Could you check a few things on this model? Use its own coordinates, in mm. Face numbers are marked on the shaded views. A direction names the side the tool comes from. Round coordinates to 2 decimals unless told otherwise and drop trailing zeros. Loops run counter-clockwise (first coordinate to the right, second up) from the corner with the lowest first, then second, coordinate; pieces in that order, holes last.
from build123d import *

# Parameters (mm, degrees)
BOSS_EXTRUDE1_DEPTH = 50
SKETCH2_W           = 7
SKETCH2_H           = 8
BOSS_EXTRUDE2_DEPTH = 50
SKETCH2_3_W         = 7
SKETCH2_3_H         = 8
BOSS_EXTRUDE3_DEPTH = 18
SKETCH3_W           = 10
SKETCH3_H           = 63
SKETCH3_W_2         = 7
SKETCH3_H_2         = 8
BOSS_EXTRUDE4_DEPTH = 82
FILLET1_R           = 5
SKETCH4_W           = 49
SKETCH4_H           = 29.5
CUT_EXTRUDE1_DEPTH  = 63
SKETCH5_W           = 29.5
SKETCH5_H           = 11
BOSS_EXTRUDE5_DEPTH = 49
CUT_EXTRUDE2_DEPTH  = 29.5
SKETCH6_R           = 1.75
CUT_EXTRUDE3_DEPTH  = 5
SKETCH6_6_R         = 0.75
CUT_EXTRUDE4_DEPTH  = 15
SKETCH8_W           = 18
SKETCH8_H           = 9.5
CUT_EXTRUDE5_DEPTH  = 40
SKETCH9_W           = 7
SKETCH9_H           = 9.5
CUT_EXTRUDE6_DEPTH  = 45
SKETCH10_W          = 10
SKETCH10_H          = 10
CUT_EXTRUDE7_DEPTH  = 29.5
SKETCH11_W          = 13
SKETCH11_H          = 48
SKETCH11_H_2        = 7
CUT_EXTRUDE8_DEPTH  = 124.13610356
SKETCH12_W          = 8
SKETCH12_H          = 10
CUT_EXTRUDE9_DEPTH  = 114.279521539
SKETCH13_W          = 10
SKETCH13_H          = 6
CUT_EXTRUDE10_DEPTH = 14
SKETCH15_W          = 14
SKETCH15_H          = 6
CUT_EXTRUDE11_DEPTH = 128.218316291
FILLET2_R           = 3


with BuildPart() as part:
    # Sketch1 → Boss-Extrude1 (new body)
    with BuildSketch(Plane.XY):
        with BuildLine():
            Line((-2.25, -8), (-4.25, -8))
            ThreePointArc((-4.25, -8), (-3.25, -8.5), (-2.25, -8))
        make_face()
        Polygon((10, -25.5), (10, 0), (0, 0), (-18, 0), (-18, -8), (0, -8), (0, -17.5), (-18, -17.5), (-18, -25.5), align=None)
    extrude(amount=BOSS_EXTRUDE1_DEPTH)

    # Sketch2 → Boss-Extrude2 (add)
    with BuildSketch(Plane(origin=(0, 0, 0), x_dir=(0, 0, -1), z_dir=(1, 0, 0))):
        Polygon((7, 0), (0, 0), (0, -8), (2.25, -8), (4.25, -8), (7, -8), align=None)
        Polygon((0, -8), (0, 0), (-10, 0), (-10, -25.5), (0, -25.5), (0, -17.5), align=None)
        with Locations((3.5, -21.5)):
            Rectangle(SKETCH2_W, SKETCH2_H)
        with BuildLine():
            Line((4.25, -8), (2.25, -8))
            ThreePointArc((2.25, -8), (3.25, -8.5), (4.25, -8))
        make_face()
    extrude(amount=BOSS_EXTRUDE2_DEPTH)

    # Sketch2<3> → Boss-Extrude3 (add)
    with BuildSketch(Plane(origin=(0, 0, 0), x_dir=(0, 0, -1), z_dir=(1, 0, 0))):
        Polygon((7, 0), (0, 0), (0, -8), (2.25, -8), (4.25, -8), (7, -8), align=None)
        with Locations((3.5, -21.5)):
            Rectangle(SKETCH2_3_W, SKETCH2_3_H)
    extrude(amount=-BOSS_EXTRUDE3_DEPTH)

    # Sketch3 → Boss-Extrude4 (add)
    with BuildSketch(Plane(origin=(50, 0, 0), x_dir=(0, 0, -1), z_dir=(1, 0, 0))):
        Polygon((36.5, -17.5), (7, -17.5), (7, -25.5), (0, -25.5), (0, -88.5), (36.5, -88.5), align=None)
        with Locations((-5, -57)):
            Rectangle(SKETCH3_W, SKETCH3_H)
        with Locations((3.5, -21.5)):
            Rectangle(SKETCH3_W_2, SKETCH3_H_2)
        with Locations((-5, -21.5)):
            Rectangle(SKETCH3_W, SKETCH3_H_2)
    extrude(amount=-BOSS_EXTRUDE4_DEPTH)

    # Fillet1
    fillet1_edges = [part.edges().sort_by_distance(p)[0] for p in [
        (-32, -17.5, -13.25),
        (-32, -53, -36.5),
        (9, -17.5, -36.5),
    ]]
    fillet(fillet1_edges, radius=FILLET1_R)

    # Sketch4 → Cut-Extrude1 (cut)
    with BuildSketch(Plane.XZ.offset(88.5)):
        with Locations((25.5, -4.75)):
            Rectangle(SKETCH4_W, SKETCH4_H)
    extrude(amount=-CUT_EXTRUDE1_DEPTH, mode=Mode.SUBTRACT)

    # Sketch5 → Boss-Extrude5 (add)
    with BuildSketch(Plane(origin=(50, 0, 0), x_dir=(0, 0, -1), z_dir=(1, 0, 0))):
        with Locations((4.75, -31)):
            Rectangle(SKETCH5_W, SKETCH5_H)
        with Locations((4.75, -83)):
            Rectangle(SKETCH5_W, SKETCH5_H)
    extrude(amount=-BOSS_EXTRUDE5_DEPTH)

    # Sketch7 → Cut-Extrude2 (cut)
    with BuildSketch(Plane.XY.offset(10)):
        Polygon((1, -36.5), (27, -36.5), (27, -26.5), (50, -26.5), (50, -88.5), (27, -88.5), (27, -77.5), (1, -77.5), align=None)
    extrude(amount=-CUT_EXTRUDE2_DEPTH, mode=Mode.SUBTRACT)

    # Sketch6 → Cut-Extrude3 (cut)
    with BuildSketch(Plane(origin=(27, 0, 0), x_dir=(0, 0, -1), z_dir=(1, 0, 0))):
        with Locations((4.25, -81.5)):
            Circle(SKETCH6_R)
        with Locations((14.25, -81.5)):
            Circle(SKETCH6_R)
        with Locations((14.25, -32.5)):
            Circle(SKETCH6_R)
        with Locations((4.25, -32.5)):
            Circle(SKETCH6_R)
    extrude(amount=-CUT_EXTRUDE3_DEPTH, mode=Mode.SUBTRACT)

    # Sketch6<6> → Cut-Extrude4 (cut)
    with BuildSketch(Plane(origin=(27, 0, 0), x_dir=(0, 0, -1), z_dir=(1, 0, 0))):
        with Locations((4.25, -81.5)):
            Circle(SKETCH6_6_R)
        with Locations((14.25, -81.5)):
            Circle(SKETCH6_6_R)
        with Locations((14.25, -32.5)):
            Circle(SKETCH6_6_R)
        with Locations((4.25, -32.5)):
            Circle(SKETCH6_6_R)
    extrude(amount=-CUT_EXTRUDE4_DEPTH, mode=Mode.SUBTRACT)

    # Sketch8 → Cut-Extrude5 (cut)
    with BuildSketch(Plane(origin=(0, 0, -7), x_dir=(-1, 0, 0), z_dir=(0, 0, -1))):
        with Locations((9, -12.75)):
            Rectangle(SKETCH8_W, SKETCH8_H)
    extrude(amount=-CUT_EXTRUDE5_DEPTH, mode=Mode.SUBTRACT)

    # Sketch9 → Cut-Extrude6 (cut)
    with BuildSketch(Plane.ZY.offset(18)):
        with Locations((-3.5, -12.75)):
            Rectangle(SKETCH9_W, SKETCH9_H)
    extrude(amount=-CUT_EXTRUDE6_DEPTH, mode=Mode.SUBTRACT)

    # Sketch10 → Cut-Extrude7 (cut)
    with BuildSketch(Plane.XY.offset(10)):
        with Locations((6, -31.5)):
            Rectangle(SKETCH10_W, SKETCH10_H)
    extrude(amount=-CUT_EXTRUDE7_DEPTH, mode=Mode.SUBTRACT)

    # Sketch11 → Cut-Extrude8 (cut, through all)
    with BuildSketch(Plane.XY.offset(-19.5)):
        with Locations((43.5, -57.5)):
            Rectangle(SKETCH11_W, SKETCH11_H)
        with Locations((43.5, -85)):
            Rectangle(SKETCH11_W, SKETCH11_H_2)
    extrude(amount=-CUT_EXTRUDE8_DEPTH, mode=Mode.SUBTRACT)

    # Sketch12 → Cut-Extrude9 (cut, through all)
    with BuildSketch(Plane.XZ.offset(88.5)):
        with Locations((-28, -31.5)):
            Rectangle(SKETCH12_W, SKETCH12_H)
    extrude(amount=-CUT_EXTRUDE9_DEPTH, mode=Mode.SUBTRACT)

    # Sketch13 → Cut-Extrude10 (cut)
    with BuildSketch(Plane.ZY.offset(32)):
        with Locations((-31.5, -20.5)):
            Rectangle(SKETCH13_W, SKETCH13_H)
    extrude(amount=-CUT_EXTRUDE10_DEPTH, mode=Mode.SUBTRACT)

    # Sketch15 → Cut-Extrude11 (cut, through all)
    with BuildSketch(Plane(origin=(0, 0, -26.5), x_dir=(-1, 0, 0), z_dir=(0, 0, -1))):
        with Locations((25, -20.5)):
            Rectangle(SKETCH15_W, SKETCH15_H)
    extrude(amount=-CUT_EXTRUDE11_DEPTH, mode=Mode.SUBTRACT)

    # Fillet2
    fillet2_edges = [part.edges().sort_by_distance(p)[0] for p in [
        (-24, -56, -26.5),
        (-24, -23.5, -31.5),
        (-28, -23.5, -26.5),
    ]]
    fillet(fillet2_edges, radius=FILLET2_R)


solid = part.part
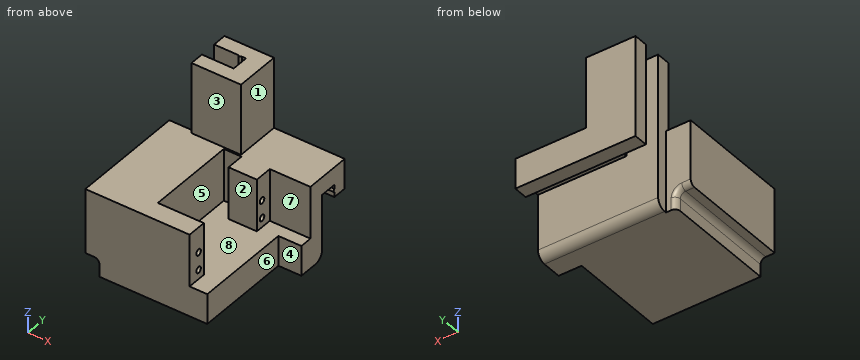
Item 1: If we section it at D-D, the plane x = 30.5: Please give me the cut outline in (y, z), then the cut area to 3 significant figures.
Results list:
outline: (-88.5, -36.5) - (-22.5, -36.5) arc R5 ccw to (-17.5, -31.5) - (-17.5, 0) - (-8, 0) - (-8, -2.25) arc R1.25 ccw to (-8, -4.25) - (-8, -7) - (0, -7) - (0, 10) - (-26.5, 10) - (-26.5, -19.5) - (-88.5, -19.5) - close
area: 1,700 mm2
Item 2: For the marked faces 1, 2, 3 and 4, which set-ups out of +Z, -Z, +X, -X, +Y, -Y let a thin tool reach every point of the face, with its end or its side?
Results list:
face 1: +Z, +X, +Y, -Y
face 2: +Z, +X
face 3: +Z, +X, -X, -Y
face 4: +Z, -Z, +X, -Y
Item 3: We'd pull the mould along Y, two halves only. Please class the marked faces 5, 6, 7 and 8: released by +Y, released by -Y, zero draft, split by the parting line, or undercut.
Results list:
face 5: undercut
face 6: zero draft
face 7: released by -Y
face 8: undercut
Item 4: If we section it at C-C, the plane z = 21.5: Please give me the cut outline in (x, y).
Results list:
outline: (-18, -25.5) - (10, -25.5) - (10, 0) - (-18, 0) - (-18, -8) - (0, -8) - (0, -17.5) - (-18, -17.5) - close
Item 5: If I drill on line 1 along Y through (x, z) = (23.25, -4.25); line 2 along Y through (x, z) = (25, -14); line 3 along Y through (x, z) = (16, -14.25), over which ranges is the centre line in solid material (lowest first)?
Results list:
line 1: y = -88.5 to -83.25, -79.75 to -77.5, -36.5 to -34.25, -30.75 to -17.5, -8 to 0
line 2: y = -88.5 to -83.23, -79.77 to -77.5, -36.5 to -34.23, -30.77 to -17.5
line 3: y = -88.5 to -82.25, -80.75 to -77.5, -36.5 to -33.25, -31.75 to -17.5
Item 6: If we section it at A-A, the plane x = -13: Please give me the cut outline in (y, z), then the cut area to 3 significant figures.
Results list:
outline: (-88.5, -36.5) - (-22.5, -36.5) arc R5 ccw to (-17.5, -31.5) - (-17.5, 50) - (-25.5, 50) - (-25.5, 10) - (-88.5, 10) - close; (-8, -7) - (0, -7) - (0, 50) - (-8, 50) - close
area: 4,070 mm2
Item 7: Will these pins go through, and if not, where does the flat tip stop? pin 1 (4 mm diameter, centred on x = 32.5, y = -5.5, fed in from -Z); pin 2 (7.5 mm diameter, centred on y = -10.5, z = 21.5, fed in from -X); pin 3 (6 mm diameter, centred on y = -58, z = 11, fed in from +X).
Results list:
pin 1: stops at z = -7
pin 2: stops at x = -18
pin 3: stops at x = 1
Item 8: If we section it at B-B, the plane y = -53.5: Please give me the cut outline in (x, z), then the cut area to 3 significant figures.
Results list:
outline: (-32, -26.5) - (-27, -26.5) arc R3 cw to (-24, -29.5) - (-24, -36.5) - (37, -36.5) - (37, -19.5) - (1, -19.5) - (1, 10) - (-32, 10) - close
area: 2,070 mm2
